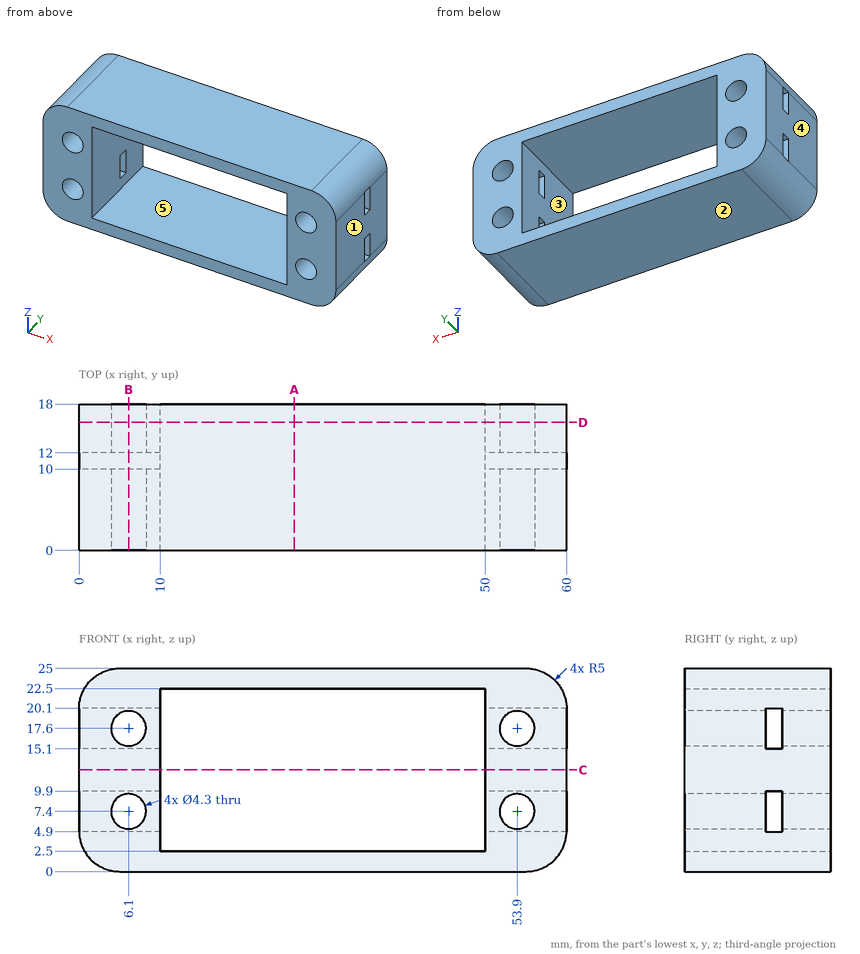
The drawing under review shows one solid part. Ordinate dimensions are in mm from its lowest x, y, z. A direction names the side the tool comes from. Give positions to 0.01 mm unless a question says otherwise; leave off trailing zeros. Loops run counter-clockwise (first coordinate to the right, second up) from the corner with the lowest first, then second, coordinate; pieces in that order, holes last. Notation, with made-up numbers: M 27,74.25 L 52,74.25 A32 cw 52,108.25 Z; hole C 74.5,-17.75 d3. An arc over 180 degrees is marked long. Return JSON: item names as keys, results as strings. Group by question number.
Item 1: For probe 1 along X at (y, z) = (7.5, 17.6); probe 2 along Z at (x, y) = (26, 6.25); probe 3 along X at (y, z) = (9, 4.75), list the stretches that pass through material, from the lowest coordinate up.
Item 2: Insertion check: pin 1 Ø5.5 at (x, z) = (6.1, 17.6) entering from -Y. The pin has a flat end and moves straight along its axis. Give the tip position at first contact, or say it passes through.
Item 3: Mouldability with a two-part tool opening along X and no side actions: class the marked faces 1, 2 and 3 as released by +X, released by -X, zero draft, split by the parting line, or undercut.
Item 4: We need section B-B (x = 6.1). Give the boundary of the cut face in (y, z).
Item 5: Tool access review of the marked faces 4 and 5: name each direction out of +Z, -Z, +X, -X, +Y, -Y from which nothing blocks a thin tool from reaching the whole face with its end or side.
Item 6: We need section C-C (z = 12.5). Give the boundary of the cut face in (x, y), and give its area (3 significant figures).
Item 7: We need section D-D (y = 15.75). Give the boundary of the cut face in (x, z).
Item 8: We need section A-A (x = 26.5). Give the boundary of the cut face in (y, z), and give its area (3 significant figures).
Output:
{
 "1": {"probe 1": "x = 0 to 3.95, 8.25 to 10, 50 to 51.75, 56.05 to 60", "probe 2": "z = 0 to 2.5, 22.5 to 25", "probe 3": "x = 0.01 to 10, 50 to 59.99"},
 "2": {"pin 1": "stops at y = 0"},
 "3": {"face 1": "released by +X", "face 2": "zero draft", "face 3": "undercut"},
 "4": {"outline": "M 0,0 L 18,0 L 18,5.25 L 12,5.25 L 12,4.9 L 10,4.9 L 10,5.25 L 0,5.25 Z; M 0,9.55 L 10,9.55 L 10,9.9 L 12,9.9 L 12,9.55 L 18,9.55 L 18,15.45 L 12,15.45 L 12,15.1 L 10,15.1 L 10,15.45 L 0,15.45 Z; M 0,19.75 L 10,19.75 L 10,20.1 L 12,20.1 L 12,19.75 L 18,19.75 L 18,25 L 0,25 Z"},
 "5": {"face 4": "+Z, -Z, -X, +Y, -Y", "face 5": "+Y, -Y"},
 "6": {"outline": "M 0,0 L 10,0 L 10,18 L 0,18 Z; M 50,0 L 60,0 L 60,18 L 50,18 Z", "area": "360 mm^2"},
 "7": {"outline": "M 0,5 A5 ccw 5,0 L 55,0 A5 ccw 60,5 L 60,20 A5 ccw 55,25 L 5,25 A5 ccw 0,20 Z; hole C 6.1,7.4 d4.3; hole C 6.1,17.6 d4.3; hole M 10,2.5 L 50,2.5 L 50,22.5 L 10,22.5 Z; hole C 53.9,7.4 d4.3; hole C 53.9,17.6 d4.3"},
 "8": {"outline": "M 0,0 L 18,0 L 18,2.5 L 0,2.5 Z; M 0,22.5 L 18,22.5 L 18,25 L 0,25 Z", "area": "90.0 mm^2"}
}
